Work out the finished part from the listing and answer in its coordinate system (mm). Coordinates: 2 decimals unless noted, no trailing zeros. Order: outer loops, then holes, each group sorted by start corner. A loop starts at its lowest first (then second) coordinate and runs counter-clockwise, first axis right, second up. Notation, with made-up numbers: (58, 58.25) -> (73, 58.25) arc R14 cw to (73, 78.25) -> close; hole circle Ø8 at (59, 6). An arc over 180 degrees is marked (long way). Answer as CSV lines item,"result". Start each with the question number.
Item 1: Straight lines are drawn through the part: L1, parallel to Y at x = 9, z = 0.3; L2, parallel to Y at x = 5, z = -1.5; L3, parallel to Z at x = -10, y = 1.75. For each, find the intervals that lie inside material, in ascending order.
Item 2: This flat-tipped pin is pushed along its axis until it touches: pin 1 Ø2 at (x, y) = (-14.5, -2) entering from +Z. Where does it stop, or does it pass through?
Item 3: Section A-A (x = 15) is taken. Write down the section's boundary in (y, z).
Solid Edge part; units mm, degrees
sketch "Sketch1" plane through (0, 0, 0) normal (1, 0, 0) x (0, 1, 0)
  circle A0 centre (0, 0) radius 3
extrude "Protrusion1" add sketch "Sketch1" along normal mid plane 40
chamfer "Chamfer_1" distance 0.5 angle 45 2 edges at (20, -3, 0) (-20, -3, 0)
sketch "Sketch2" plane through (0, 0, 0) normal (1, 0, 0) x (0, 1, 0)
  circle A0 centre (0, 3) radius 0.2
extrude "ExtrudedCutout_1" cut sketch "Sketch2" along normal mid plane 49.1824
pattern_circular "Pattern1" count 6 over 360 about axis through (0, 0, 0) along (-1, 0, 0) of "ExtrudedCutout_1"
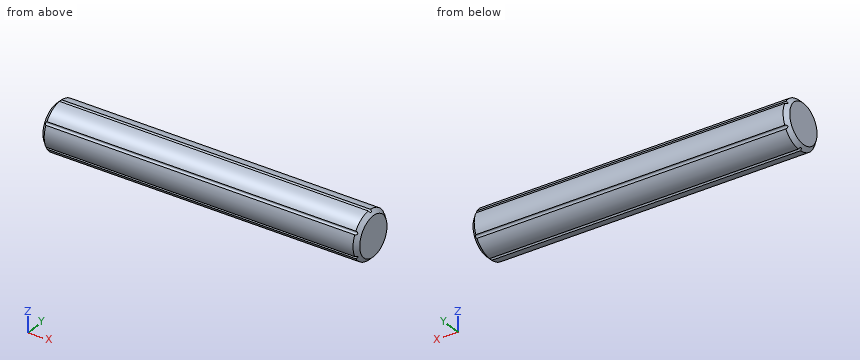
Checked values:
1,L1,"y = -2.98 to 2.98"
1,L2,"y = -2.4 to 2.4"
1,L3,"z = -2.44 to 2.44"
2,pin 1,"stops at z = 2.83"
3,outline,"(-2.69, -1.32) arc R0.2 cw to (-2.49, -1.67) arc R3 ccw to (-0.2, -2.99) arc R0.2 cw to (0.2, -2.99) arc R3 ccw to (2.49, -1.67) arc R0.2 cw to (2.69, -1.32) arc R3 ccw to (2.69, 1.32) arc R0.2 cw to (2.49, 1.67) arc R3 ccw to (0.2, 2.99) arc R0.2 cw to (-0.2, 2.99) arc R3 ccw to (-2.49, 1.67) arc R0.2 cw to (-2.69, 1.32) arc R3 ccw to start"
